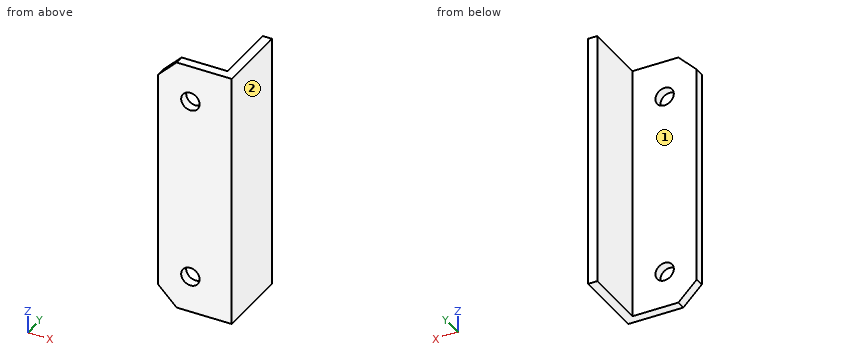
from build123d import *

# Parameters (mm, degrees)
EXTRUDE_THIN1_DEPTH      = 70
EXTRUDE_THIN1_DEPTH_BACK = 70
CHAMFER1_SIZE            = 10
SKETCH2_R                = 5
CUT_EXTRUDE1_DEPTH       = 10


with BuildPart() as part:
    # Sketch1 → Extrude-Thin1 (new, two sides: drawn at the far end of the back side and taken through both)
    with BuildSketch(Plane.XY.offset(-EXTRUDE_THIN1_DEPTH_BACK)):
        Polygon((-40, 0), (0, 0), (0, 40), (-5, 40), (-5, 5), (-40, 5), align=None)
    extrude(amount=EXTRUDE_THIN1_DEPTH + EXTRUDE_THIN1_DEPTH_BACK)

    # Chamfer1
    chamfer1_edges = [part.edges().sort_by_distance(p)[0] for p in [
        (-40, 2.5, 70),
        (-40, 2.5, -70),
    ]]
    chamfer(chamfer1_edges, length=CHAMFER1_SIZE)

    # Sketch2 → Cut-Extrude1 (cut)
    with BuildSketch(Plane(origin=(0, 5, 0), x_dir=(1, 0, 0), z_dir=(0, 1, 0))):
        with Locations(Location((-22.5, 50, 0), (0, 0, 270))):
            Circle(SKETCH2_R)
        with Locations(Location((-22.5, -50, 0), (0, 0, 270))):
            Circle(SKETCH2_R)
    extrude(amount=-CUT_EXTRUDE1_DEPTH, mode=Mode.SUBTRACT)


solid = part.part
Geometry check sheet. Reference: the model listing, model coordinates, mm. Face numbers are marked on the shaded views. A direction names the side the tool comes from. Give positions to 0.01 mm unless a question says otherwise; leave off trailing zeros. Order: outer loops, then holes, each group sorted by start corner. A loop starts at its lowest first (then second) coordinate and runs counter-clockwise, first axis right, second up. Notation, with made-up numbers: (38.25, 53.25) - (66.25, 53.25) arc R27 ccw to (66.25, 74.25) - close; hole circle Ø3 at (-31.5, -10.75). An arc over 180 degrees is marked (long way). Answer as a JSON object with one key per item and string values.
(1) Cross-section at D-D (z = -0.5). Record the cut outline in (x, y), then the cut area to 3 significant figures.
Report:
{"outline": "(-40, 0) - (0, 0) - (0, 40) - (-5, 40) - (-5, 5) - (-40, 5) - close", "area": "375 mm^2"}
(2) Tool access check on the marked faces 1 and 2. Record the directions out of +Z, -Z, +X, -X, +Y, -Y that give a thin tool (end or side, any length) a straight path to the whole face; none if there is none.
Report:
{"face 1": "+Z, -Z, -X, +Y", "face 2": "+Z, -Z, +X, +Y, -Y"}
(3) Cross-section at C-C (y = 3). Record the cut outline in (x, z), then the cut area to 3 significant figures.
Report:
{"outline": "(-40, -60) - (-30, -70) - (0, -70) - (0, 70) - (-30, 70) - (-40, 60) - close; hole circle Ø10 at (-22.5, -50); hole circle Ø10 at (-22.5, 50)", "area": "5,340 mm^2"}
(4) Cross-section at A-A (z = -50). Record the cut outline in (x, y).
Report:
{"outline": "(-40, 0) - (-27.5, 0) - (-27.5, 5) - (-40, 5) - close; (-17.5, 0) - (0, 0) - (0, 40) - (-5, 40) - (-5, 5) - (-17.5, 5) - close"}
(5) Material ranges on line 1 (Z direction, x = -22, y = 3); line 2 (X direction, y = 2.95, z = 50); line 3 (Y direction, x = -23.5, z = 0.5), recorded low to high.
Report:
{"line 1": "-70 to -54.97, -45.03 to 45.03, 54.97 to 70", "line 2": "-40 to -27.5, -17.5 to 0", "line 3": "0 to 5"}
(6) Cross-section at B-B (x = -22.5). Record the cut outline in (y, z), then the cut area to 3 significant figures.
Report:
{"outline": "(0, -70) - (5, -70) - (5, -55) - (0, -55) - close; (0, -45) - (5, -45) - (5, 45) - (0, 45) - close; (0, 55) - (5, 55) - (5, 70) - (0, 70) - close", "area": "600 mm^2"}
(7) Depth check by flat-ended pin: pin 1 Ø10.5 at (y, z) = (26, -9.5) entering from -X; pin 2 Ø16 at (x, z) = (-22.5, 50) entering from +Y. Enter the tip coordinate at first touch or a pass-through.
Report:
{"pin 1": "x = -5", "pin 2": "y = 5"}
